Here's how the part is built. I have some questions about the finished solid (model axes, mm). A direction names the side the tool comes from. Give positions to 0.01 mm unless a question says otherwise; leave off trailing zeros. Write each loop counter-clockwise with the first axis right and the second up, starting at its lowest first coordinate (ties: lowest second). Pieces come first, ordered by that corner, then holes. Notation, with made-up numbers: M -9.5,12.25 L 0.5,12.25 A20 cw 0.5,45.25 Z; hole C 64,-13.5 d2. An arc over 180 degrees is marked long. Answer as CSV lines item,"result". Start each with the question number.
Q1. Suppose I cut it at D-D (x = 61). Write out the boundary of the cut face in (y, z), then the cut area to 3 significant figures.
Q2. Thinking about a two-plate mould opening in X: for faces 4 (the cylindrical face through (-11.5, -22.2, 62.3)), 5 (the flat face through (-1, -26, 45)), 6 (the cylindrical face through (74, 28, 8)), 7 (the cylindrical face through (-6.92, 13.31, 50.28)), which applies, +X half, -X half, draft (parallel to the pull), parting line (faces both ways), or undercut?
Q3. Suppose I cut it at A-A (z = 10). Write out the boundary of the cut face in (x, y), then the cut area to 3 significant figures.
Q4. For pin 1 (12 mm diameter, centred on x = -50.5, y = -11.5, fed in from +Z); pin 2 (8.5 mm diameter, centred on x = 63.5, y = 0, fed in from +Z); pin 3 (13 mm diameter, centred on y = 6.5, z = 28.5, fed in from -X), each with a flat end and sliding along its axis, tell me the tip position at first contact or that it passes through.
Q5. If I drill on line 1 along Y through (x, z) = (61, 4); line 2 along X through (y, z) = (0, 74); line 3 along X through (y, z) = (15, 8), over which ranges is the centre line in solid material (lowest first)?
Q6. Suppose I cut it at B-B (x = 0). Write out the boundary of the cut face in (y, z).
Q7. Suppose I cut it at C-C (z = 20). Write out the boundary of the cut face in (x, y).
Q8. On a 3-axis mill with a long thin cutter (end or side, diameter ignored), from which of +Z, -Z, +X, -X, +Y, -Y can I reach the whole of each face in a straight line? I mean faces 1 (the flat face through (31, 6, 21)), 2 (the flat face through (61, 0, 15)), 3 (the flat face through (-35, -18, 14)). Say none if no direction works.
Autodesk Fusion 360 part; units mm, degrees
sketch "Sketch2" plane through (0, 0, 0) normal (0, 0, 1) x (1, 0, 0)
  line L0 (-75, 30) -> (75, 30)
  line L1 (75, 30) -> (75, -30)
  line L2 (75, -30) -> (-75, -30)
  line L3 (-75, -30) -> (-75, 30)
  point P0 (-75, 0)
  point P1 (0, 30)
  point P2 (-75, 30)
  point P3 (0, -30)
  point P4 (-75, -30)
  point P5 (-75, 0)
  point P6 (75, 0)
  point P7 (75, 80)
  point P8 (-75, 80)
  point P9 (75, 30)
  point P10 (-75, 30)
  point P11 (-75, -30)
  point P12 (75, -30)
  point P13 (-45, 30)
  point P14 (-45, -30)
  point P15 (75, -30)
  point P16 (75, 30)
  point P17 (45, 45)
  point P18 (-45, 45)
  point P19 (-45, 15)
  point P20 (-75, 15)
  point P21 (-75, 0)
  point P22 (-35, 0)
  point P23 (-35, 30)
  point P24 (35, 30)
  point P25 (35, 0)
  point P26 (75, 0)
  point P27 (75, 15)
  point P28 (45, 15)
  point P29 (-75, 30)
  point P30 (-75, -30)
  point P31 (75, -30)
  point P32 (75, 30)
  point P33 (30, 28)
  point P34 (-30, 28)
  point P35 (-30, 0)
  point P36 (30, 0)
  point P37 (-35, 31)
  point P38 (-35, 0)
  point P39 (-20, 0)
  point P40 (-20, 31)
  point P41 (30, 28)
  point P42 (-30, 28)
  point P43 (-30, 0)
  point P44 (30, 0)
  dimension "d3" = 150
extrude "Extrude1" add sketch "Sketch2" along normal blind 80 makes body 1
sketch "Sketch3" plane through (0, 30, 0) normal (0, 1, 0) x (-1, 0, 0)
  line L0 (-75, 0) -> (75, 0)
  line L1 (75, 0) -> (75, 80)
  line L2 (75, 80) -> (-75, 80)
  line L3 (-75, 80) -> (-75, 0)
  line L4 (-35, 0) -> (35, 0)
  line L5 (35, 0) -> (35, 30)
  line L6 (35, 30) -> (-35, 30)
  line L7 (-35, 30) -> (-35, 0)
  point P0 (-35, 0)
  point P1 (35, 0)
  dimension "d6" = 30
extrude "Extrude2" cut sketch "Sketch3" against normal blind 95 contours L0 L4 L5 L6 L7 bodies 1
sketch "Sketch4" plane through (0, 0, 80) normal (0, 0, 1) x (-1, 0, 0)
  line L0 (75, 30) -> (-75, 30)
  line L1 (-75, 30) -> (-75, -30)
  line L2 (-75, -30) -> (75, -30)
  line L3 (75, -30) -> (75, 30)
  line L4 (-75, 30) -> (-45, 30)
  line L5 (-45, 30) -> (-45, -30)
  line L6 (-45, -30) -> (-75, -30)
  line L7 (-75, -30) -> (-75, 30)
  dimension "d9" = 30
  dimension "d10" = 60
extrude "Extrude3" cut sketch "Sketch4" against normal blind 65 contours L0 L1 L2 L4 L5 L6 L7 bodies 1
sketch "Sketch5" plane through (0, 0, 80) normal (0, 0, 1) x (-1, 0, 0)
  line L0 (-45, 30) -> (-45, -30)
  line L1 (-45, -30) -> (75, -30)
  line L2 (75, -30) -> (75, 30)
  line L3 (75, 30) -> (-45, 30)
  line L4 (45, 30) -> (75, 30)
  line L5 (75, 30) -> (75, -30)
  line L6 (75, -30) -> (45, -30)
  line L7 (45, -30) -> (45, 30)
extrude "Extrude4" cut sketch "Sketch5" against normal blind 65 contours L1 L2 L3 L4 L5 L6 L7 bodies 1
extrude "Extrude5" cut 1 faces at (-15, 10, 80) along direction (0, 0, -1) blind 35 on bodies 1 bodies 1
sketch "Sketch6" plane through (0, 30, 0) normal (0, 1, 0) x (-1, 0, 0)
  line L0 (45, 45) -> (-45, 45)
  line L1 (-45, 45) -> (-45, 15)
  line L2 (-45, 15) -> (-75, 15)
  line L3 (-75, 15) -> (-75, 0)
  line L4 (-75, 0) -> (-35, 0)
  line L5 (-35, 0) -> (-35, 30)
  line L6 (-35, 30) -> (35, 30)
  line L7 (35, 30) -> (35, 0)
  line L8 (35, 0) -> (75, 0)
  line L9 (75, 0) -> (75, 15)
  line L10 (75, 15) -> (45, 15)
  line L11 (45, 15) -> (45, 45)
sketch "Sketch7" plane through (0, 30, 0) normal (0, 1, 0) x (-1, 0, 0)
fillet "Fillet1" radius 2 1 edges at (-45, 0, 45) on bodies 1
fillet "Fillet2" radius 2 1 edges at (45, 0, 45) on bodies 1
fillet "Fillet3" radius 2 1 edges at (45, 0, 15) on bodies 1
fillet "Fillet4" radius 2 1 edges at (-45, 0, 15) on bodies 1
sketch "Sketch8" plane through (0, 0, 15) normal (0, 0, 1) x (-1, 0, 0)
  line L0 (-47, -30) -> (-47, 30)
  line L1 (-47, 30) -> (-75, 30)
  line L2 (-75, 30) -> (-75, -30)
  line L3 (-75, -30) -> (-47, -30)
  line L4 (-61, 30) -> (-61, -30)
  line L5 (-75, 0) -> (-47, 0)
  circle A0 centre (-61, 15) radius 6
  circle A1 centre (-61, -15) radius 6
  dimension "d25" = 12
  dimension "d26" = 12
extrude "Extrude6" cut sketch "Sketch8" against normal blind 14 contours L4 A1 | L4 A1 bodies 1
extrude "Extrude7" cut 1 faces at (63.268, 17.2246, 1) along direction (0, 0, -1) blind 16 on bodies 1 bodies 1
extrude "Extrude8" cut sketch "Sketch8" against normal blind 21 contours L4 A0 | L4 A0 bodies 1
sketch "Sketch9" plane through (0, 0, 15) normal (0, 0, 1) x (-1, 0, 0)
  line L0 (47, 30) -> (47, -30)
  line L1 (47, -30) -> (75, -30)
  line L2 (75, -30) -> (75, 30)
  line L3 (75, 30) -> (47, 30)
  circle A0 centre (75, 0) radius 7
  dimension "d33" = 14
extrude "Extrude9" cut sketch "Sketch9" against normal blind 34 contours L2 A0 picked at (77.2388, 0.6574) bodies 1
sketch "Sketch10" plane through (0, 0, 15) normal (0, 0, 1) x (-1, 0, 0)
  circle A0 centre (-70, 25) radius 5
  circle A1 centre (-70, -25) radius 5
  arc A2 (-75, -25) -> (-70, -30) centre (-72.5, -27.5) ccw
  arc A3 (-70, 30) -> (-75, 25) centre (-72.5, 27.5) ccw
  point P0 (-72.5, 30)
  point P1 (-75, 27.5)
  point P2 (-75, 30)
  point P3 (-70, 30)
  point P4 (-75, 25)
  point P5 (-70, -30)
  point P6 (-75, -25)
  dimension "d37" = 10
  dimension "d38" = 10
extrude "Extrude10" cut sketch "Sketch10" against normal blind 17 contours A0 A3 bodies 1
extrude "Extrude11" cut sketch "Sketch10" against normal blind 23 contours A1 A2 bodies 1
sketch "Sketch11" plane through (0, 0, 45) normal (0, 0, 1) x (-1, 0, 0)
  line L0 (-43, 30) -> (-43, -30)
  line L1 (-43, -30) -> (43, -30)
  line L2 (43, -30) -> (43, 30)
  line L3 (43, 30) -> (-43, 30)
sketch "Sketch12" plane through (0, 0, 45) normal (0, 0, 1) x (-1, 0, 0)
sketch "Sketch13" plane through (0, 0, 45) normal (0, 0, 1) x (-1, 0, 0)
  circle A0 centre (0, 0) radius 25
  point P0 (0, 30)
  point P1 (75, 30)
  point P2 (0, -30)
  point P3 (-45, 0)
  point P4 (47, 0)
  dimension "d43" = 50
extrude "Extrude12" add sketch "Sketch13" along normal blind 35 bodies 1
sketch "Sketch14" plane through (0, 0, 80) normal (0, 0, 1) x (-1, 0, 0)
  circle A0 centre (0, 0) radius 25
  circle A1 centre (0, 0) radius 20
  dimension "d46" = 40
extrude "Extrude13" cut sketch "Sketch14" against normal blind 10 contours A1 bodies 1
sketch "Sketch15" plane through (0, 0, 70) normal (0, 0, 1) x (-1, 0, 0)
  circle A0 centre (0, 0) radius 20
  circle A1 centre (0, 0) radius 15
  dimension "d49" = 30
extrude "Extrude14" cut sketch "Sketch15" against normal blind 25 contours A1 bodies 1
sketch "Sketch16" plane through (0, 0, 0) normal (0, 1, 0) x (1, 0, 0)
  line L0 (0, -80) -> (0, -59)
  circle A0 centre (0, -59) radius 5
  point P0 (0, -80)
  dimension "d52" = 21
  dimension "d53" = 10
extrude "Extrude15" cut sketch "Sketch16" along normal blind -40 and the other way blind -40 bodies 1
fillet "Fillet5" radius 2 1 edges at (-35, 0, 30) on bodies 1
fillet "Fillet6" radius 2 1 edges at (35, 0, 30) on bodies 1
sketch "Sketch17" plane through (-35, 0, 0) normal (1, 0, 0) x (0, 1, 0)
  line L0 (30, 28) -> (-30, 28)
  line L1 (-30, 28) -> (-30, 0)
  line L2 (-30, 0) -> (30, 0)
  line L3 (30, 0) -> (30, 28)
  line L4 (-6, 0) -> (6, 0)
  line L5 (-6, 0) -> (-6, 31)
  line L6 (-6, 31) -> (6, 31)
  line L7 (6, 31) -> (6, 0)
extrude "Extrude16" add sketch "Sketch17" along normal blind 15 separate body contours L0 L2 L4 L5 L7 | L0 L5 L6 L7 makes body 2
sketch "Sketch18" plane through (0, -6, 0) normal (0, -1, 0) x (1, 0, 0)
  line L0 (-35, 31) -> (-35, 0)
  line L1 (-35, 0) -> (-20, 0)
  line L2 (-20, 0) -> (-20, 31)
  line L3 (-20, 31) -> (-35, 31)
  line L4 (-35, 0) -> (-20, 30)
  line L5 (-35, 0) -> (-20, 0)
  line L6 (-20, 0) -> (-20, 30)
extrude "Extrude17" cut sketch "Sketch18" against normal blind 54 contours L1 L2 L4 L5 L6 bodies 2
sketch "Sketch19" plane through (35, 0, 0) normal (-1, 0, 0) x (0, -1, 0)
  line L0 (30, 28) -> (-30, 28)
  line L1 (-30, 28) -> (-30, 0)
  line L2 (-30, 0) -> (30, 0)
  line L3 (30, 0) -> (30, 28)
copy_body "CopyPasteBodies1" bodies 2 makes body 3
move_body "Move1" bodies 3 to x (-1, 0, 0) y (0, -1, 0) z (0, 0, 1) at (-27, -12, 0)
move_body "Move2" bodies 3 to x (1, 0, 0) y (0, 1, 0) z (0, 0, 1) at (27, 12, 0)
sketch "Sketch20" plane through (0, 0, 0) normal (0, 1, 0) x (1, 0, 0)
extrude "Extrude18" cut sketch "Sketch15" against normal blind 45 contours A1 bodies 1
combine "Combine1" operation add target body 1 tool bodies 2 3
Resolved:
1,outline,"M -30,0 L -21,0 L -21,15 L -30,15 Z; M -9,0 L 9,0 L 9,15 L -9,15 Z; M 21,0 L 30,0 L 30,15 L 21,15 Z"
1,area,"540 mm^2"
2,face 4,"parting line"
2,face 5,"draft"
2,face 6,"+X half"
2,face 7,"undercut"
3,outline,"M -75,-30 L -35,-30 L -35,-6 L -30,-6 L -30,6 L -35,6 L -35,30 L -75,30 Z; M 30,-6 L 35,-6 L 35,-30 L 70,-30 A5 ccw 75,-25 L 75,25 A5 ccw 70,30 L 35,30 L 35,6 L 30,6 Z; hole C 61,-15 d12; hole C 61,15 d12"
3,area,"4,680 mm^2"
4,pin 1,"z = 44.32"
4,pin 2,"z = 15"
4,pin 3,"x = -45"
5,line 1,"-30 to -21, -9 to 9, 21 to 30"
5,line 2,"-25 to -20, 20 to 25"
5,line 3,"-75 to -35, 35 to 55, 67 to 75"
6,outline,"M -30,30 L -15,30 L -15,54 L -25,54 L -25,45 L -30,45 Z; M -25,64 L -15,64 L -15,70 L -20,70 L -20,80 L -25,80 Z; M 15,30 L 30,30 L 30,45 L 25,45 L 25,54 L 15,54 Z; M 15,64 L 25,64 L 25,80 L 20,80 L 20,70 L 15,70 Z"
7,outline,"M -45,-30 L -35,-30 L -35,-6 L -25,-6 L -25,6 L -35,6 L -35,30 L -45,30 Z; M 25,-6 L 35,-6 L 35,-30 L 45,-30 L 45,30 L 35,30 L 35,6 L 25,6 Z"
8,face 1,"-Z, +Y"
8,face 2,"+Z, +X, +Y, -Y"
8,face 3,"-Z, -Y"
